For this review, take the finished solid that the model builds, in its own axes (mm). Face numbers are marked on the shaded views. A direction names the side the tool comes from. Give positions to 0.01 mm unless a question says otherwise; leave off trailing zeros. Loops run counter-clockwise (first coordinate to the right, second up) from the corner with the lowest first, then second, coordinate; pieces in that order, holes last. Notation, with made-up numbers: M -4.5,0.25 L 51.5,0.25 A24 ccw 51.5,22.25 Z; hole C 83,-6.5 d6. An arc over 180 degrees is marked long. Use CSV: the item, a comma, the result in double quotes. Start each with the question number.
1. Take a section at D-D, the plane z = 9. Write out the cut boundary in (x, y).
2. Take a section at A-A, the plane z = 3.5. Write out the cut boundary in (x, y).
3. The part is to be moulded in two halves that separate along X. For the marked faces 4, 5 and 6, say which applies: pulls with the +X half, pulls with the -X half, needs draft (parallel to the pull), parting line crosses it, or undercut.
4. Tool access review of the marked faces 1, 2 and 3: name each direction out of +Z, -Z, +X, -X, +Y, -Y from which nothing blocks a thin tool from reaching the whole face with its end or side.
5. Take a section at B-B, the plane x = -12.55. Write out the cut boundary in (y, z).
6. Insertion check: P1, Ø1.3, axis at y = 15.5, z = 11, coming from the -X side; P2, Ø1.5, axis at x = -11, y = 13, coming from the +Z side; P3, Ø6, axis at x = 10.5, y = 2.5, coming from the -Z side; P4, Ø0.8, axis at y = 16.5, z = 12.5, coming from the +X side. Each pin has a flat end and moves straight along its axis. Give the tip position at first contact, or say it passes through.
7. To check wall thickness, follow line 1 (Y direction, x = 8, z = 9); line 2 (Y direction, x = -12.5, z = 11); line 3 (X direction, y = 15.5, z = 13.25). State the ranges of each line that lie inside material, in increasing order. Write a range as [from, to].
8. Take a section at C-C, the plane y = 7. Write out the cut boundary in (x, z).
from build123d import *

# Parameters (mm, degrees)
ESQUISSE1_R             = 1.4
BOSS_EXTRU_1_DEPTH      = 16
ESQUISSE2_W             = 15.7
ESQUISSE2_H             = 16
BOSS_EXTRU_2_DEPTH      = 15
ESQUISSE3_R             = 4
ENL_V_MAT_EXTRU_1_DEPTH = 15
ESQUISSE4_W             = 21
ESQUISSE4_H             = 8
ENL_V_MAT_EXTRU_2_DEPTH = 21
ESQUISSE5_R             = 1.4
ENL_V_MAT_EXTRU_3_DEPTH = 21
ESQUISSE6_W             = 18.213974707
ESQUISSE6_H             = 12
ENL_V_MAT_EXTRU_4_DEPTH = 10
ESQUISSE7_R             = 1.2
ENL_V_MAT_EXTRU_5_DEPTH = 24.669600757
BOSS_EXTRU_3_DEPTH      = 8


with BuildPart() as part:
    # Esquisse1 → Boss.-Extru.1 (new body)
    with BuildSketch(Plane.XY):
        Polygon((15.5, 10), (-15.5, 10), (-15.5, 0), (-10.5, 0), (-10.5, 5), (10.5, 5), (10.5, 0), (15.5, 0), align=None)
        with Locations((12.55, 3.5)):
            Circle(ESQUISSE1_R, mode=Mode.SUBTRACT)
        with Locations(Location((-12.55, 3.5, 0), (0, 0, 180))):
            Circle(ESQUISSE1_R, mode=Mode.SUBTRACT)
    extrude(amount=BOSS_EXTRU_1_DEPTH)

    # Esquisse2 → Boss.-Extru.2 (add)
    with BuildSketch(Plane(origin=(0, 10, 0), x_dir=(1, 0, 0), z_dir=(0, 1, 0))):
        with Locations((0, -8)):
            Rectangle(ESQUISSE2_W, ESQUISSE2_H)
    extrude(amount=BOSS_EXTRU_2_DEPTH)

    # Esquisse3 → Enlèv. mat.-Extru.1 (cut)
    with BuildSketch(Plane.XY.offset(16)):
        with Locations((0, 17.5)):
            Circle(ESQUISSE3_R)
    extrude(amount=-ENL_V_MAT_EXTRU_1_DEPTH, mode=Mode.SUBTRACT)

    # Esquisse4 → Enlèv. mat.-Extru.2 (cut)
    with BuildSketch(Plane.XZ.offset(-5)):
        with Locations((0, 4)):
            Rectangle(ESQUISSE4_W, ESQUISSE4_H)
    extrude(amount=-ENL_V_MAT_EXTRU_2_DEPTH, mode=Mode.SUBTRACT)

    # Esquisse5 → Enlèv. mat.-Extru.3 (cut)
    with BuildSketch(Plane.ZY.offset(7.85)):
        with Locations((12, 17.5)):
            Circle(ESQUISSE5_R)
    extrude(amount=-ENL_V_MAT_EXTRU_3_DEPTH, mode=Mode.SUBTRACT)

    # Esquisse6 → Enlèv. mat.-Extru.4 (cut)
    with BuildSketch(Plane.XY.offset(16)):
        with Locations((-1.256987354, 19)):
            Rectangle(ESQUISSE6_W, ESQUISSE6_H)
    extrude(amount=-ENL_V_MAT_EXTRU_4_DEPTH, mode=Mode.SUBTRACT)

    # Esquisse7 → Enlèv. mat.-Extru.5 (cut, through all)
    with BuildSketch(Plane.XZ.offset(-5)):
        with Locations(Location((0, 12, 0), (0, 0, 270))):
            Circle(ESQUISSE7_R)
    extrude(amount=-ENL_V_MAT_EXTRU_5_DEPTH, mode=Mode.SUBTRACT)

    # Esquisse8 → Boss.-Extru.3 (add)
    with BuildSketch(Plane.XY.offset(16)):
        Polygon((-7.85, 13), (-7.85, 15), (-10.35, 15), (-10.35, 17.5), (-4.85, 17.5), (-4.85, 13), align=None)
        Polygon((4.85, 13), (7.85, 13), (7.85, 15), (10.35, 15), (10.35, 17.5), (4.85, 17.5), align=None)
    extrude(amount=-BOSS_EXTRU_3_DEPTH)


solid = part.part
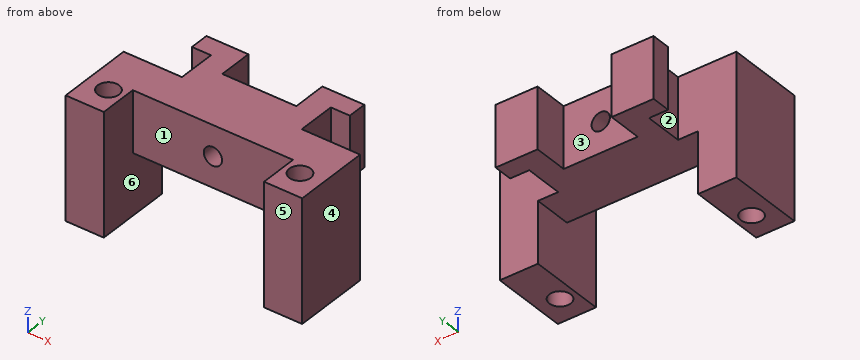
Result set:
1,outline,"M -15.5,0 L -10.5,0 L -10.5,5 L 10.5,5 L 10.5,0 L 15.5,0 L 15.5,10 L 7.85,10 L 7.85,15 L 10.35,15 L 10.35,17.5 L 4.85,17.5 L 4.85,13 L -4.85,13 L -4.85,17.5 L -10.35,17.5 L -10.35,15 L -7.85,15 L -7.85,10 L -15.5,10 Z; hole C -12.55,3.5 d2.8; hole C 12.55,3.5 d2.8"
2,outline,"M -15.5,0 L -10.5,0 L -10.5,10 L -15.5,10 Z; M 10.5,0 L 15.5,0 L 15.5,10 L 10.5,10 Z; hole C -12.55,3.5 d2.8; hole C 12.55,3.5 d2.8"
3,face 4,"pulls with the +X half"
3,face 5,"needs draft"
3,face 6,"undercut"
4,face 1,"+Z, -Z, -Y"
4,face 2,"+Z, -Z, -X"
4,face 3,"+Z, -Z, +Y"
5,outline,"M 0,0 L 2.1,0 L 2.1,16 L 0,16 Z; M 4.9,0 L 10,0 L 10,16 L 4.9,16 Z"
6,P1,"x = -10.35"
6,P2,"through"
6,P3,"z = 0"
6,P4,"x = 10.35"
7,line 1,"[5, 10], [15, 17.5]"
7,line 2,"[0, 2.1], [4.9, 10]"
7,line 3,"[-10.35, -4.85], [4.85, 10.35]"
8,outline,"M -15.5,0 L -10.5,0 L -10.5,8 L 10.5,8 L 10.5,0 L 15.5,0 L 15.5,16 L -15.5,16 Z; hole C 0,12 d2.4"
